Check sheet for the drawn part. Datum: minimum x, y, z corner. Units: mm. A direction names the side the tool comes from. Round coordinates to 2 decimals unless told otherwise and drop trailing zeros. Order: outer loops, then holes, each group sorted by start corner. A loop starts at its lowest first (then second) coordinate and runs counter-clockwise, first axis right, second up. Notation, with made-up numbers: M 24.25,2 L 53.25,2 A31 cw 53.25,41 Z; hole C 87.5,22 d3. An arc over 180 degrees is marked long. Write item = value, one per line. Start each with the question number.
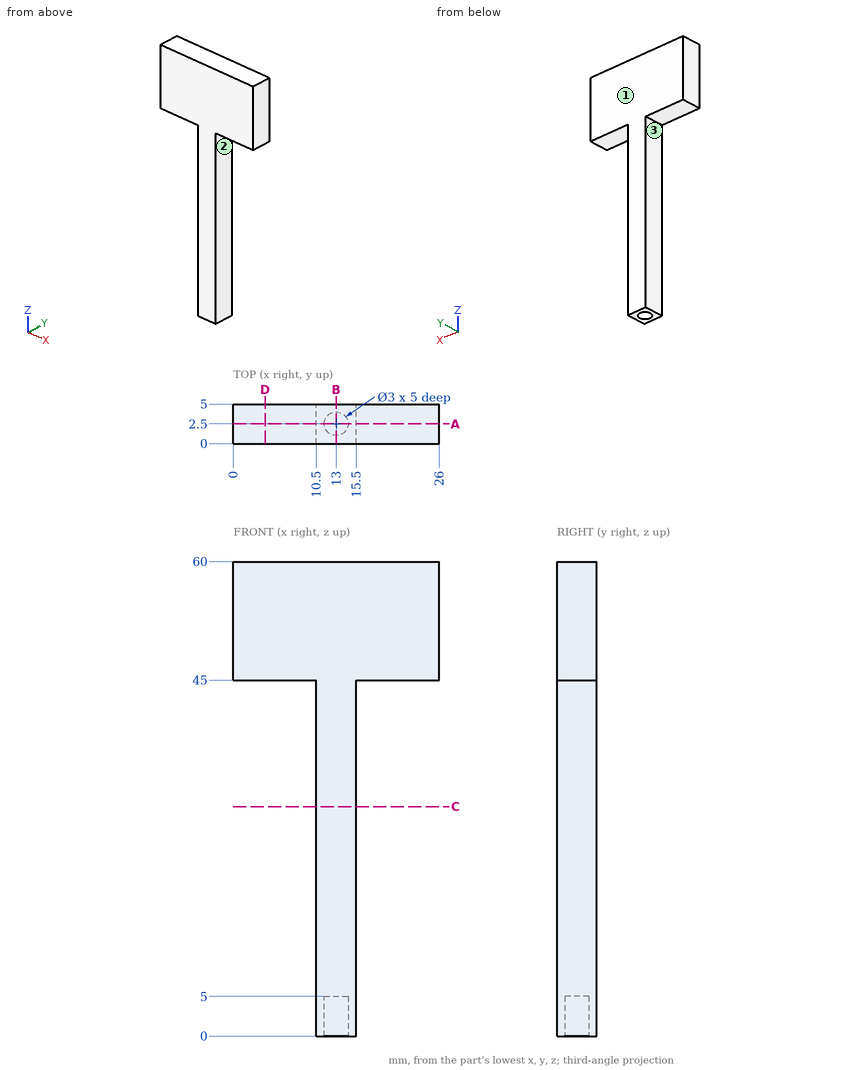
1) Cross-section at C-C, the plane z = 29. Enter the section's corners in (x, y), then the cut area to 3 significant figures.
2) Cross-section at A-A, the plane y = 2.5. Enter the section's corners in (x, z), then the cut area to 3 significant figures.
3) Cross-section at B-B, the plane x = 13. Enter the section's corners in (y, z).
4) Scan lines: probe 1 along Y at (x, z) = (13, 2.15); probe 2 along X at (y, z) = (2.3, 4.5); probe 3 along Z at (x, y) = (3.5, 3.15). Record each from-to range of solid material in increasing order.
5) Access from +Z, -Z, +X, -X, +Y, -Y to the whole of each face (thin tool, end or side, straight path). Record for the marked faces 1, 2 and 3.
6) Gauge pin test, flat ends, axial feed: P1, Ø1.5, axis at y = 2, z = 22.5, coming from the -X side; P2, Ø1.5, axis at x = 13.5, y = 3, coming from the -Z side; P3, Ø3, axis at x = 18, y = 2.5, coming from the -Z side. Record the tip position at first contact, or that the pin passes through.
7) Cross-section at D-D, the plane x = 4. Enter the section's corners in (y, z), then the cut area to 3 significant figures.
Geometry results:
q1.outline = M 10.5,0 L 15.5,0 L 15.5,5 L 10.5,5 Z
q1.area = 25.0 mm^2
q2.outline = M 0,45 L 10.5,45 L 10.5,0 L 11.5,0 L 11.5,5 L 14.5,5 L 14.5,0 L 15.5,0 L 15.5,45 L 26,45 L 26,60 L 0,60 Z
q2.area = 600 mm^2
q3.outline = M 0,0 L 1,0 L 1,5 L 4,5 L 4,0 L 5,0 L 5,60 L 0,60 Z
q4.probe_1 = 0 to 1, 4 to 5
q4.probe_2 = 10.5 to 11.51, 14.49 to 15.5
q4.probe_3 = 45 to 60
q5.face_1 = +Z, -Z, +X, -X, +Y
q5.face_2 = -Z, +X, +Y, -Y
q5.face_3 = -Z, -X, +Y, -Y
q6.P1 = 10.5
q6.P2 = 5
q6.P3 = 45
q7.outline = M 0,45 L 5,45 L 5,60 L 0,60 Z
q7.area = 75.0 mm^2
